```python
from build123d import *

# Parameters (mm, degrees)
EXTRUDE_1_DEPTH      = 13
EXTRUDE_1_DEPTH_BACK = 13
SKETCH_2_R           = 5
CUT_EXTRUDE_1_DEPTH  = 38.322915213
SKETCH_3_R           = 1.6
CUT_EXTRUDE_2_DEPTH  = 37.783148315
EXTRUDE_START        = 3
SKETCH_4_W           = 18
SKETCH_4_H           = 26
SKETCH_4_R           = 1.6
EXTRUDE_2_DEPTH      = 3
EXTRUDE_START_2      = 2
SKETCH_5_W           = 26
SKETCH_5_H           = 25
SKETCH_5_R           = 5
EXTRUDE_3_DEPTH      = 2
SKETCH_6_W           = 14
SKETCH_6_H           = 5
EXTRUDE_4_DEPTH      = 8
CHAMFER_1_SIZE       = 10
FILLET_1_R           = 3
EXTRUDE_5_REACH      = 36.554
SKETCH_7_W           = 16
SKETCH_7_H           = 2
FILLET_2_R           = 15
FILLET_3_R           = 2
FILLET_4_R           = 1.6


with BuildPart() as part:
    # 草图1 → 凸台-拉伸1 (new, two sides: drawn at the far end of the back side and taken through both)
    with BuildSketch(Plane.XY.offset(-EXTRUDE_1_DEPTH_BACK)):
        Polygon((0, 30), (0, 0), (20, 0), (20, 2), (2, 2), (2, 30), align=None)
    extrude(amount=EXTRUDE_1_DEPTH + EXTRUDE_1_DEPTH_BACK)

    # 草图2 → 切除-拉伸1 (cut, through all)
    with BuildSketch(Plane(origin=(2, 0, 0), x_dir=(0, 0, -1), z_dir=(1, 0, 0))):
        with Locations((0, 22)):
            Circle(SKETCH_2_R)
    extrude(amount=-CUT_EXTRUDE_1_DEPTH, mode=Mode.SUBTRACT)

    # 草图3 → 切除-拉伸2 (cut, through all)
    with BuildSketch(Plane(origin=(0, 2, 0), x_dir=(1, 0, 0), z_dir=(0, 1, 0))):
        with Locations(Location((10, 6, 0), (0, 0, 270))):
            Circle(SKETCH_3_R)
        with Locations(Location((10, -6, 0), (0, 0, 90))):
            Circle(SKETCH_3_R)
    extrude(amount=-CUT_EXTRUDE_2_DEPTH, mode=Mode.SUBTRACT)

    # 草图4 → 凸台-拉伸2 (add)
    with BuildSketch(Plane(origin=(0, 2, 0), x_dir=(1, 0, 0), z_dir=(0, 1, 0)).offset(EXTRUDE_START)):
        with Locations((11, 0)):
            Rectangle(SKETCH_4_W, SKETCH_4_H)
        with Locations(Location((10, -6, 0), (0, 0, 270))):
            Circle(SKETCH_4_R, mode=Mode.SUBTRACT)
        with Locations(Location((10, 6, 0), (0, 0, 270))):
            Circle(SKETCH_4_R, mode=Mode.SUBTRACT)
    extrude(amount=-EXTRUDE_2_DEPTH)

    # 草图5 → 凸台-拉伸3 (add)
    with BuildSketch(Plane(origin=(2, 0, 0), x_dir=(0, 0, -1), z_dir=(1, 0, 0)).offset(EXTRUDE_START_2)):
        with Locations((0, 17.5)):
            Rectangle(SKETCH_5_W, SKETCH_5_H)
        with Locations((0, 22)):
            Circle(SKETCH_5_R, mode=Mode.SUBTRACT)
    extrude(amount=-EXTRUDE_3_DEPTH)

    # 草图6 → 凸台-拉伸4 (add)
    with BuildSketch(Plane(origin=(0, 5, 0), x_dir=(1, 0, 0), z_dir=(0, 1, 0))):
        with Locations((11, 0)):
            Rectangle(SKETCH_6_W, SKETCH_6_H)
    extrude(amount=EXTRUDE_4_DEPTH)

    # 倒角1
    # the kernel refuses this chamfer: 10 mm, written as the material it takes off along each edge
    with BuildSketch(Plane(origin=(18, 13, -28.21682988), x_dir=(-0.9996219169112968, 0.027495876610586317, 0), z_dir=(0, 0, 1))) as chamfer_1_piece_1_section:
        Polygon((CHAMFER_1_SIZE * 0.999621916911, CHAMFER_1_SIZE * 0.0274958766106), (-CHAMFER_1_SIZE * 0.0274958766106, CHAMFER_1_SIZE * 0.999621916911), (0, 0), align=None)
    chamfer_1_piece_1 = extrude(amount=56.433659759, mode=Mode.PRIVATE)
    chamfer_1_piece_1 = split(chamfer_1_piece_1, bisect_by=Plane(origin=(14.542815877, 5, 0), z_dir=(0, 1, 0)), keep=Keep.TOP, mode=Mode.PRIVATE)
    add(chamfer_1_piece_1, mode=Mode.SUBTRACT)

    # 圆角1
    fillet_1_edges = [part.edges().sort_by_distance(p)[0] for p in [
        (4, 5, 7.75),
        (4, 5, -7.75),
    ]]
    fillet(fillet_1_edges, radius=FILLET_1_R)

    # 凸台-拉伸5: up to this face of the body (flat: up to its plane)
    extrude_5_end = Plane(part.part.faces().sort_by_distance((2, 30, 0))[0])
    # 草图7 → 凸台-拉伸5 (add, up to the picked face)
    with BuildSketch(Plane(origin=(0, 5, 0), x_dir=(1, 0, 0), z_dir=(0, 1, 0)), mode=Mode.PRIVATE) as extrude_5_sk1:
        with Locations((12, 12)):
            Rectangle(SKETCH_7_W, SKETCH_7_H)
    extrude_5_tool1 = split(extrude(extrude_5_sk1.sketch, amount=EXTRUDE_5_REACH, mode=Mode.PRIVATE), bisect_by=extrude_5_end, keep=Keep.BOTH, mode=Mode.PRIVATE)
    # 草图7 → 凸台-拉伸5 (add, up to the picked face)
    with BuildSketch(Plane(origin=(0, 5, 0), x_dir=(1, 0, 0), z_dir=(0, 1, 0)), mode=Mode.PRIVATE) as extrude_5_sk2:
        with Locations((12, -12)):
            Rectangle(SKETCH_7_W, SKETCH_7_H)
    extrude_5_tool2 = split(extrude(extrude_5_sk2.sketch, amount=EXTRUDE_5_REACH, mode=Mode.PRIVATE), bisect_by=extrude_5_end, keep=Keep.BOTH, mode=Mode.PRIVATE)
    add(extrude_5_tool1.solids().sort_by(Axis((12, 5, -12), (0, 1, 0)))[0])
    add(extrude_5_tool2.solids().sort_by(Axis((12, 5, 12), (0, 1, 0)))[0])

    # 圆角2
    fillet_2_edges = [part.edges().sort_by_distance(p)[0] for p in [
        (20, 30, -12),
        (20, 30, 12),
    ]]
    fillet(fillet_2_edges, radius=FILLET_2_R)

    # 圆角3
    fillet_3_edges = [part.edges().sort_by_distance(p)[0] for p in [
        (13.5, 5, 11),
        (4.878679656, 5.878679656, 11),
        (13.5, 5, -11),
        (4.878679656, 5.878679656, -11),
        (16, 5, 0),
        (4, 19, 11),
        (4, 19, -11),
    ]]
    fillet(fillet_3_edges, radius=FILLET_3_R)

    # 圆角4
    fillet_4_edges = [part.edges().sort_by_distance(p)[0] for p in [
        (4, 13, 0),
        (8, 13, 0),
    ]]
    fillet(fillet_4_edges, radius=FILLET_4_R)


solid = part.part
```
Part model, mm, in its own coordinate system. A direction names the side the tool comes from. Give positions to 0.01 mm unless a question says otherwise; leave off trailing zeros. Write each loop counter-clockwise with the first axis right and the second up, starting at its lowest first coordinate (ties: lowest second). Pieces come first, ordered by that corner, then holes. Notation, with made-up numbers: M 58.25,20 L 91.25,20 A23 ccw 91.25,42 Z; hole C -36.75,49.5 d3. An arc over 180 degrees is marked long. Use CSV: the item, a comma, the result in double quotes.
Item 1: Drill centre lines: probe 1 along X at (y, z) = (3.25, -6); probe 2 along Z at (x, y) = (16, 12.5); probe 3 along Y at (x, z) = (1.4, 0). Where is each one in solid material? Low to high.
Taken from the geometry:
probe 1,"x = 0 to 8.4, 11.6 to 20"
probe 2,"z = -13 to -11, 11 to 13"
probe 3,"y = 0 to 17, 27 to 30"
Item 2: Slice it at B-B on y = 25.5. Write the cut outline in (x, z), plus the area to 3 significant figures.
Taken from the geometry:
outline,"M 0,-13 L 15.71,-13 L 15.71,-11 L 6,-11 A2 cw 4,-9 L 4,-3.57 L 0,-3.57 Z; M 0,3.57 L 4,3.57 L 4,9 A2 cw 6,11 L 15.71,11 L 15.71,13 L 0,13 Z"
area,"124 mm²"
Item 3: Slice it at D-D on y = 10.5. Write the cut outline in (x, z), plus the area to 3 significant figures.
Taken from the geometry:
outline,"M 0,-13 L 20,-13 L 20,-11 L 6,-11 A2 cw 4,-9 L 4,-2.5 L 10.5,-2.5 L 10.5,2.5 L 4,2.5 L 4,9 A2 cw 6,11 L 20,11 L 20,13 L 0,13 Z"
area,"202 mm²"
Item 4: Pull direction Y, two halves, no side cores. Call faces 3 (the face through (2.03, 17.12, 1.08)), 4 (the face through (9, 9, -2.5)), 5 (the face through (7.94, 12.88, 0.04)), 6 (the face through (10, 0, 0)): +Y half, -Y half, draft (parallel to the pull), parting line (faces both ways), or undercut.
Taken from the geometry:
face 3,"undercut"
face 4,"draft"
face 5,"+Y half"
face 6,"-Y half"
Item 5: Slice it at A-A on z = 6. Write the cut outline in (x, y), plus the area to 3 significant figures.
Taken from the geometry:
outline,"M 0,0 L 8.4,0 L 8.4,5 L 7,5 A3 cw 4,8 L 4,30 L 0,30 Z; M 11.6,0 L 20,0 L 20,5 L 11.6,5 Z"
area,"186 mm²"
Item 6: Slice it at C-C on x = 10. Write the cut outline in (y, z).
Taken from the geometry:
outline,"M 0,-13 L 29.14,-13 L 29.14,-11 L 7,-11 A2 cw 5,-9 L 5,-7.6 L 0,-7.6 Z; M 0,-4.4 L 5,-4.4 L 5,-2.5 L 11,-2.5 L 11,2.5 L 5,2.5 L 5,4.4 L 0,4.4 Z; M 0,7.6 L 5,7.6 L 5,9 A2 cw 7,11 L 29.14,11 L 29.14,13 L 0,13 Z"
Item 7: Pin check, flat tips, straight feed: P1, Ø0.9, axis at x = 6.5, z = 0.5, coming from the +Y side; P2, Ø4, axis at x = 15, z = 2, coming from the +Y side; P3, Ø6, axis at x = 17, z = 6.5, coming from the +Y side. Stop position of each tip, or through.
Taken from the geometry:
P1,"stops at y = 13"
P2,"stops at y = 8"
P3,"stops at y = 5.06"
Item 8: Which spindle directions (+Z, -Z, +X, -X, +Y, -Y) get a long thin tool onto all of the face, cutting with end or side? Do faces 1 (the face through (4, 16.7, 0.1)), 2 (the face through (10, 15, 13)). Say none if no direction does.
Taken from the geometry:
face 1,"+X, +Y"
face 2,"+Z, +X, -X, +Y, -Y"
